```python
from build123d import *

# Parameters (mm, degrees)
SKETCH1_W           = 50.8
SKETCH1_H           = 50.8
SKETCH1_R           = 6.5
SKETCH1_R_2         = 1.5
BOSS_EXTRUDE1_DEPTH = 3.175
SKETCH2_W           = 50.8
SKETCH2_H           = 3.175
BOSS_EXTRUDE2_DEPTH = 44.45
SKETCH3_R           = 3.175
CUT_EXTRUDE1_DEPTH  = 4.175


with BuildPart() as part:
    # Sketch1 → Boss-Extrude1 (new body)
    with BuildSketch(Plane.XY):
        with Locations((25.4, 25.4)):
            Rectangle(SKETCH1_W, SKETCH1_H)
        with Locations((25.4, 35.575)):
            Circle(SKETCH1_R, mode=Mode.SUBTRACT)
        with Locations((9.9, 28.575)):
            Circle(SKETCH1_R_2, mode=Mode.SUBTRACT)
        with Locations((40.9, 28.575)):
            Circle(SKETCH1_R_2, mode=Mode.SUBTRACT)
        with Locations((33.15, 15.151606241)):
            Circle(SKETCH1_R_2, mode=Mode.SUBTRACT)
        with Locations((17.65, 15.151606241)):
            Circle(SKETCH1_R_2, mode=Mode.SUBTRACT)
        with Locations((17.65, 41.998393759)):
            Circle(SKETCH1_R_2, mode=Mode.SUBTRACT)
        with Locations((33.15, 41.998393759)):
            Circle(SKETCH1_R_2, mode=Mode.SUBTRACT)
    extrude(amount=BOSS_EXTRUDE1_DEPTH)

    # Sketch2 → Boss-Extrude2 (add)
    with BuildSketch(Plane.XY.offset(3.175)):
        with Locations((25.4, 1.5875)):
            Rectangle(SKETCH2_W, SKETCH2_H)
    extrude(amount=BOSS_EXTRUDE2_DEPTH)

    # Sketch3 → Cut-Extrude1 (cut, through all)
    with BuildSketch(Plane(origin=(0, 3.175, 0), x_dir=(1, 0, 0), z_dir=(0, 1, 0))):
        with Locations((25.4, -15.875)):
            Circle(SKETCH3_R)
        with Locations((25.4, -34.925)):
            Circle(SKETCH3_R)
    extrude(amount=-CUT_EXTRUDE1_DEPTH, mode=Mode.SUBTRACT)


solid = part.part
```
Build history of the part. All positions in model axes, mm. A direction names the side the tool comes from. Give positions to 0.01 mm unless a question says otherwise; leave off trailing zeros. Loops run counter-clockwise (first coordinate to the right, second up) from the corner with the lowest first, then second, coordinate; pieces in that order, holes last. Notation, with made-up numbers: (74, -29) - (101, -29) arc R24 cw to (101, -16) - close; hole circle Ø8 at (81.25, 23). An arc over 180 degrees is marked (long way). Use a Markdown table: item, result.
(1) Wall check: line 1 along Y through (x, z) = (17.65, 2.05); line 2 along Z through (x, y) = (25, 1) (3 decimals); line 3 along Y through (x, z) = (15, 5.5) (3 decimals). Give the ranges that are in metal, low to high.
Taken from the geometry:
| item | result |
|---|---|
| line 1 | 0 to 13.65, 16.65 to 40.5, 43.5 to 50.8 |
| line 2 | 0 to 12.725, 19.025 to 31.775, 38.075 to 47.625 |
| line 3 | 0 to 3.175 |
(2) Drop flat-ended pins along their axis: pin 1 Ø5 at (x, y) = (17.65, 42) entering from +Z (3 decimals); pin 2 Ø8 at (x, z) = (35.5, 24.5) entering from +Y (3 decimals). Give the stop position or say it passes through.
Taken from the geometry:
| item | result |
|---|---|
| pin 1 | z = 3.175 |
| pin 2 | y = 3.175 |
(3) Which spindle directions (+Z, -Z, +X, -X, +Y, -Y) get a long thin tool onto all of the face, cutting with end or side? Do faces 4 (the face through (25, 3.175, 25)), 5 (the face through (33.842, 40.668, 1.565)). Say none if no direction does.
Taken from the geometry:
| item | result |
|---|---|
| face 4 | +Z, +X, -X, +Y |
| face 5 | +Z, -Z |
(4) Band-saw the part on A-A (x = 17.65). Give the cut face in (y, z) (3 decimals).
Taken from the geometry:
| item | result |
|---|---|
| outline | (0, 0) - (13.652, 0) - (13.652, 3.175) - (3.175, 3.175) - (3.175, 47.625) - (0, 47.625) - close; (16.652, 0) - (40.498, 0) - (40.498, 3.175) - (16.652, 3.175) - close; (43.498, 0) - (50.8, 0) - (50.8, 3.175) - (43.498, 3.175) - close |
(5) Band-saw the part on C-C (z = 17). Give the cut face in (x, y) (3 decimals).
Taken from the geometry:
| item | result |
|---|---|
| outline | (0, 0) - (22.431, 0) - (22.431, 3.175) - (0, 3.175) - close; (28.369, 0) - (50.8, 0) - (50.8, 3.175) - (28.369, 3.175) - close |
(6) Band-saw the part on B-B (x = 9.9). Give the cut face in (y, z) (3 decimals).
Taken from the geometry:
| item | result |
|---|---|
| outline | (0, 0) - (27.075, 0) - (27.075, 3.175) - (3.175, 3.175) - (3.175, 47.625) - (0, 47.625) - close; (30.075, 0) - (50.8, 0) - (50.8, 3.175) - (30.075, 3.175) - close |
(7) Pull direction X, two halves, no side cores. Call faces 1 (the face through (25, 50.8, 2)), 2 (the face through (19.08, 15.6, 1.57)), 3 (the face through (50.8, 14, 3)): +X half, -X half, draft (parallel to the pull), parting line (faces both ways), or undercut.
Taken from the geometry:
| item | result |
|---|---|
| face 1 | draft |
| face 2 | undercut |
| face 3 | +X half |
(8) Band-saw the part on D-D (y = 5). Give the cut face in (x, z) (3 decimals), and give its area (3 significant figures).
Taken from the geometry:
| item | result |
|---|---|
| outline | (0, 0) - (50.8, 0) - (50.8, 3.175) - (0, 3.175) - close |
| area | 161 mm2 |
